```python
from build123d import *

# Parameters (mm, degrees)
SKETCH1_R           = 30
BOSS_EXTRUDE1_DEPTH = 25


with BuildPart() as part:
    # Sketch1 → Boss-Extrude1 (new body)
    with BuildSketch(Plane(origin=(0, 0, 0), x_dir=(1, 0, 0), z_dir=(0, 1, 0))):
        with BuildLine():
            Line((-63.8, 107.8), (-107.8, 107.8))
            Line((-107.8, 107.8), (-107.8, 63.8))
            ThreePointArc((-107.8, 63.8), (-98.288961426, 35.388965946), (-73, 19.323003766))
            Line((-73, 19.323003766), (-73, -19.323003766))
            ThreePointArc((-73, -19.323003766), (-98.288961426, -35.388965946), (-107.8, -63.8))
            Line((-107.8, -63.8), (-107.8, -107.8))
            Line((-107.8, -107.8), (-63.8, -107.8))
            ThreePointArc((-63.8, -107.8), (-28.653661458, -91.775146025), (-19.03272249, -54.365273115))
            ThreePointArc((-19.03272249, -54.365273115), (-15.743256927, -44.108614607), (-5.551800988, -40.62237691))
            ThreePointArc((-5.551800988, -40.62237691), (0, -41), (5.551800988, -40.62237691))
            ThreePointArc((5.551800988, -40.62237691), (15.743256927, -44.108614607), (19.03272249, -54.365273115))
            ThreePointArc((19.03272249, -54.365273115), (28.653661458, -91.775146025), (63.8, -107.8))
            Line((63.8, -107.8), (107.8, -107.8))
            Line((107.8, -107.8), (107.8, -63.8))
            ThreePointArc((107.8, -63.8), (98.288961426, -35.388965946), (73, -19.323003766))
            Line((73, -19.323003766), (73, 19.323003766))
            ThreePointArc((73, 19.323003766), (98.288961426, 35.388965946), (107.8, 63.8))
            Line((107.8, 63.8), (107.8, 107.8))
            Line((107.8, 107.8), (63.8, 107.8))
            ThreePointArc((63.8, 107.8), (28.653661458, 91.775146025), (19.03272249, 54.365273115))
            ThreePointArc((19.03272249, 54.365273115), (15.743256927, 44.108614607), (5.551800988, 40.62237691))
            ThreePointArc((5.551800988, 40.62237691), (0, 41), (-5.551800988, 40.62237691))
            ThreePointArc((-5.551800988, 40.62237691), (-15.743256927, 44.108614607), (-19.03272249, 54.365273115))
            ThreePointArc((-19.03272249, 54.365273115), (-28.653661458, 91.775146025), (-63.8, 107.8))
        make_face()
        with BuildLine():
            Line((-94.245355165, -95.115537993), (-95.5, -95.1))
            Line((-95.5, -95.1), (-95.5, -93.845258955))
            Line((-95.5, -93.845258955), (-95.5, -63))
            ThreePointArc((-95.5, -63), (-39.877175844, -40.161764449), (-63.40246135, -95.497507979))
            Line((-63.40246135, -95.497507979), (-94.245355165, -95.115537993))
        make_face(mode=Mode.SUBTRACT)
        with BuildLine():
            Line((95.5, -93.845258955), (95.5, -95.1))
            Line((95.5, -95.1), (94.245355165, -95.115537993))
            Line((94.245355165, -95.115537993), (63.40246135, -95.497507979))
            ThreePointArc((63.40246135, -95.497507979), (39.877175844, -40.161764449), (95.5, -63))
            Line((95.5, -63), (95.5, -93.845258955))
        make_face(mode=Mode.SUBTRACT)
        with Locations(Location((0, 0, 0), (0, 0, 270))):
            Circle(SKETCH1_R, mode=Mode.SUBTRACT)
        with BuildLine():
            Line((-95.5, 93.845258955), (-95.5, 95.1))
            Line((-95.5, 95.1), (-94.245355165, 95.115537993))
            Line((-94.245355165, 95.115537993), (-63.40246135, 95.497507979))
            ThreePointArc((-63.40246135, 95.497507979), (-39.877175844, 40.161764449), (-95.5, 63))
            Line((-95.5, 63), (-95.5, 93.845258955))
        make_face(mode=Mode.SUBTRACT)
        with BuildLine():
            Line((94.245355165, 95.115537993), (95.5, 95.1))
            Line((95.5, 95.1), (95.5, 93.845258955))
            Line((95.5, 93.845258955), (95.5, 63))
            ThreePointArc((95.5, 63), (39.877175844, 40.161764449), (63.40246135, 95.497507979))
            Line((63.40246135, 95.497507979), (94.245355165, 95.115537993))
        make_face(mode=Mode.SUBTRACT)
    extrude(amount=BOSS_EXTRUDE1_DEPTH)


solid = part.part
```
Work out the finished part from the listing and answer in its coordinate system (mm). A direction names the side the tool comes from. Round coordinates to 2 decimals unless told otherwise and drop trailing zeros. Write each loop counter-clockwise with the first axis right and the second up, starting at its lowest first coordinate (ties: lowest second). Pieces come first, ordered by that corner, then holes. Notation, with made-up numbers: (42.5, 43) -> (91.5, 43) arc R30 ccw to (91.5, 65) -> close; hole circle Ø1 at (4, 81). An arc over 180 degrees is marked (long way). Write each question's results on one line, items separated by ' | '.
1) Flat-ended cylindrical pins translate along their axes: pin 1 (5 mm diameter, centred on x = 75.5, y = 11, fed in from +Z); pin 2 (7.5 mm diameter, centred on y = 18, z = -78, fed in from -X); pin 3 (8 mm diameter, centred on x = -22.5, y = 9, fed in from -Z). Find the tip coordinate at first contact, or state that the pin passes through.
Findings:
pin 1: stops at z = 107.8 | pin 2: stops at x = -107.8 | pin 3: stops at z = -88.99
2) The part is cut by section A-A (z = 0). Write down the section's boundary in (x, y), and give its area (3 significant figures).
Findings:
outline: (-73, 0) -> (-30, 0) -> (-30, 25) -> (-73, 25) -> close; (30, 0) -> (73, 0) -> (73, 25) -> (30, 25) -> close | area: 2,150 mm²
3) The part is cut by section B-B (x = 60). Write down the section's boundary in (y, z), and give its area (3 significant figures).
Findings:
outline: (0, -107.71) -> (25, -107.71) -> (25, -95.36) -> (0, -95.36) -> close; (0, -30.64) -> (25, -30.64) -> (25, 30.64) -> (0, 30.64) -> close; (0, 95.36) -> (25, 95.36) -> (25, 107.71) -> (0, 107.71) -> close | area: 2,150 mm²
4) Which of the six approach directions +Z, -Z, +X, -X, +Y, -Y give full straight-line access (tool end or side, diameter ignored) to faces 1 (the cylindrical face through (98.02, 12.32, -35.05)), 2 (the cylindrical face through (-39.135, 12.325, -40.939)), 3 (the cylindrical face through (-98.551, 12.325, -35.727))?
Findings:
face 1: +X, +Y, -Y | face 2: +Y, -Y | face 3: -X, +Y, -Y
5) Consider line 1 along X through (y, z) = (15.5, -63); line 2 along Z through (x, y) = (63, 10.5); line 3 along X through (y, z) = (23.75, -83.5). Determine where each line is inside the solid, lowest interval first. Write a range as [from, to].
Findings:
line 1: x = [-107.81, -95.5], [-30.5, -18.19], [18.19, 30.5], [95.5, 107.81] | line 2: z = [-107.81, -95.5], [-30.5, 30.5], [95.5, 107.81] | line 3: x = [-107.8, -95.5], [-37.78, -23.16], [23.16, 37.78], [95.5, 107.8]
6) The part is cut by section D-D (x = -91). Write down the section's boundary in (y, z), and give its area (3 significant figures).
Findings:
outline: (0, -107.8) -> (25, -107.8) -> (25, -95.16) -> (0, -95.16) -> close; (0, -46.5) -> (25, -46.5) -> (25, -28.02) -> (0, -28.02) -> close; (0, 28.02) -> (25, 28.02) -> (25, 46.5) -> (0, 46.5) -> close; (0, 95.16) -> (25, 95.16) -> (25, 107.8) -> (0, 107.8) -> close | area: 1,560 mm²
7) For a pull along X with two mould halves and no side action, classify faces 4 (the cylindrical face through (-40.645, 12.325, 39.41)), 5 (the flat face through (95.5, 12, 79)), 6 (the cylindrical face through (98.551, 12.325, 35.727)), 7 (the flat face through (-107.8, 12, 85)) as +X half, -X half, draft (parallel to the pull), parting line (faces both ways), or undercut.
Findings:
face 4: undercut | face 5: undercut | face 6: +X half | face 7: -X half
8) The part is cut by section C-C (z = -70). Write down the section's boundary in (x, y), and give its area (3 significant figures).
Findings:
outline: (-107.8, 0) -> (-95.5, 0) -> (-95.5, 25) -> (-107.8, 25) -> close; (-31.26, 0) -> (-18.74, 0) -> (-18.74, 25) -> (-31.26, 25) -> close; (18.74, 0) -> (31.26, 0) -> (31.26, 25) -> (18.74, 25) -> close; (95.5, 0) -> (107.8, 0) -> (107.8, 25) -> (95.5, 25) -> close | area: 1,240 mm²
